```python
from build123d import *

# Parameters (mm, degrees)
SKETCH1_R           = 5
BOSS_EXTRUDE2_DEPTH = 10


with BuildPart() as part:
    # Sketch1 → Boss-Extrude2 (new body)
    with BuildSketch(Plane(origin=(0, 0, 0), x_dir=(1, 0, 0), z_dir=(0, 1, 0))):
        with BuildLine():
            ThreePointArc((0, 60), (-42.426406871, 42.426406871), (-60, 0))
            ThreePointArc((-60, 0), (-42.426406871, -42.426406871), (0, -60))
            ThreePointArc((0, -60), (42.426406871, -42.426406871), (60, 0))
            ThreePointArc((60, 0), (42.426406871, 42.426406871), (0, 60))
        make_face()
        with Locations(Location((-25, 43.301270189, 0), (0, 0, 270))):
            Circle(SKETCH1_R, mode=Mode.SUBTRACT)
        with Locations(Location((-17.5, 30.310889132, 0), (0, 0, 270))):
            Circle(SKETCH1_R, mode=Mode.SUBTRACT)
        with Locations(Location((-10, 17.320508076, 0), (0, 0, 270))):
            Circle(SKETCH1_R, mode=Mode.SUBTRACT)
        with Locations(Location((25, 43.301270189, 0), (0, 0, 270))):
            Circle(SKETCH1_R, mode=Mode.SUBTRACT)
        with Locations(Location((17.5, 30.310889132, 0), (0, 0, 270))):
            Circle(SKETCH1_R, mode=Mode.SUBTRACT)
        with Locations(Location((10, 17.320508076, 0), (0, 0, 270))):
            Circle(SKETCH1_R, mode=Mode.SUBTRACT)
        with Locations(Location((50, 0, 0), (0, 0, 270))):
            Circle(SKETCH1_R, mode=Mode.SUBTRACT)
        with Locations(Location((35, 0, 0), (0, 0, 270))):
            Circle(SKETCH1_R, mode=Mode.SUBTRACT)
        with Locations(Location((20, 0, 0), (0, 0, 270))):
            Circle(SKETCH1_R, mode=Mode.SUBTRACT)
        with Locations(Location((25, -43.301270189, 0), (0, 0, 270))):
            Circle(SKETCH1_R, mode=Mode.SUBTRACT)
        with Locations(Location((17.5, -30.310889132, 0), (0, 0, 270))):
            Circle(SKETCH1_R, mode=Mode.SUBTRACT)
        with Locations(Location((10, -17.320508076, 0), (0, 0, 270))):
            Circle(SKETCH1_R, mode=Mode.SUBTRACT)
        with Locations(Location((-25, -43.301270189, 0), (0, 0, 270))):
            Circle(SKETCH1_R, mode=Mode.SUBTRACT)
        with Locations(Location((-17.5, -30.310889132, 0), (0, 0, 270))):
            Circle(SKETCH1_R, mode=Mode.SUBTRACT)
        with Locations(Location((-10, -17.320508076, 0), (0, 0, 270))):
            Circle(SKETCH1_R, mode=Mode.SUBTRACT)
        with Locations(Location((-50, 0, 0), (0, 0, 270))):
            Circle(SKETCH1_R, mode=Mode.SUBTRACT)
        with Locations(Location((-35, 0, 0), (0, 0, 270))):
            Circle(SKETCH1_R, mode=Mode.SUBTRACT)
        with Locations(Location((-20, 0, 0), (0, 0, 270))):
            Circle(SKETCH1_R, mode=Mode.SUBTRACT)
        with BuildLine():
            ThreePointArc((0, 10), (-7.071067812, 7.071067812), (-10, 0))
            ThreePointArc((-10, 0), (-7.071067812, -7.071067812), (0, -10))
            ThreePointArc((0, -10), (7.071067812, -7.071067812), (10, 0))
            ThreePointArc((10, 0), (7.071067812, 7.071067812), (0, 10))
        make_face(mode=Mode.SUBTRACT)
    extrude(amount=BOSS_EXTRUDE2_DEPTH)


solid = part.part
```
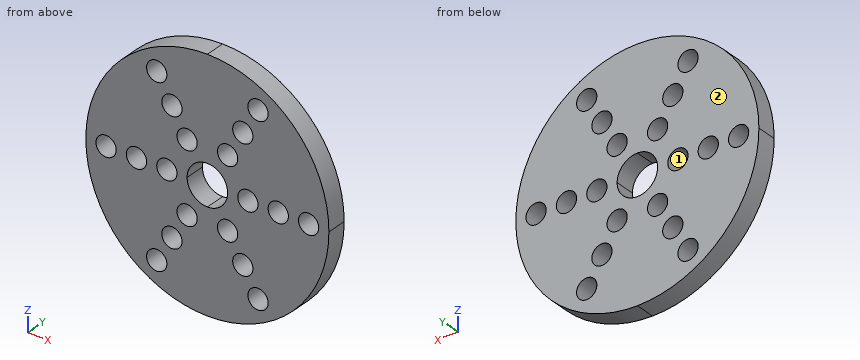
The model under review builds one solid part; all positions refer to its coordinate system, in mm. Face numbers are marked on the shaded views. Coordinates: 2 decimals unless noted, no trailing zeros. Write each loop counter-clockwise with the first axis right and the second up, starting at its lowest first coordinate (ties: lowest second). Pieces come first, ordered by that corner, then holes.
1) We need section C-C on x = -35. State the section outline as (y, z) points.
2) We need section D-D on x = 50. State the section outline as (y, z) points, then the cut area to 3 significant figures.
3) The part is to be moulded in two halves that separate along Z. For the marked faces 1 and 2, say which applies: pulls with the +Z half, pulls with the -Z half, needs draft (parallel to the pull), parting line crosses it, or undercut.
4) Clearance check with flat-ended pins moving along their axes: pin 1 Ø2 at (x, y) = (-15.5, 8) entering from -Z; pin 2 Ø4 at (x, y) = (-16.5, 6) entering from +Z; pin 3 Ø8 at (x, z) = (10, -17.32) entering from -Y; pin 4 Ø5 at (y, z) = (4.5, -47) entering from -X. State where each tip first meets the part, or that it passes through.
5) We need section B-B on z = -16.5. State the section outline as (x, y) points, then the cut area to 3 significant figures.
6) We need section A-A on y = 1.5. Count the separate pieces of the cut face and the enclosed holes in it, then the cut area to 3 significant figures.
7) To check wall thickness, follow probe 1 along X at (y, z) = (4, 41); probe 2 along Z at (x, y) = (29, 1.5); probe 3 along Z at (x, y) = (-28, 6.5). State the ranges of each line that lie inside material, in increasing order.
Answer list:
1. outline: (0, -48.73) - (10, -48.73) - (10, -5) - (0, -5) - close; (0, 5) - (10, 5) - (10, 48.73) - (0, 48.73) - close
2. outline: (0, -33.17) - (10, -33.17) - (10, -5) - (0, -5) - close; (0, 5) - (10, 5) - (10, 33.17) - (0, 33.17) - close
2. area: 563 mm2
3. face 1: undercut
3. face 2: needs draft
4. pin 1: stops at z = -58.22
4. pin 2: stops at z = 58.22
4. pin 3: passes through
4. pin 4: stops at x = -40.25
5. outline: (-57.69, 0) - (-14.93, 0) - (-14.93, 10) - (-57.69, 10) - close; (-5.07, 0) - (5.07, 0) - (5.07, 10) - (-5.07, 10) - close; (14.93, 0) - (57.69, 0) - (57.69, 10) - (14.93, 10) - close
5. area: 956 mm2
6. separate pieces: 1
6. enclosed holes: 19
6. area: 9,580 mm2
7. probe 1: x = -43.81 to -29.44, -20.56 to 20.56, 29.44 to 43.81
7. probe 2: z = -52.53 to -46.3, -40.3 to 40.3, 46.3 to 52.53
7. probe 3: z = -53.07 to -47.3, -39.3 to 39.3, 47.3 to 53.07
